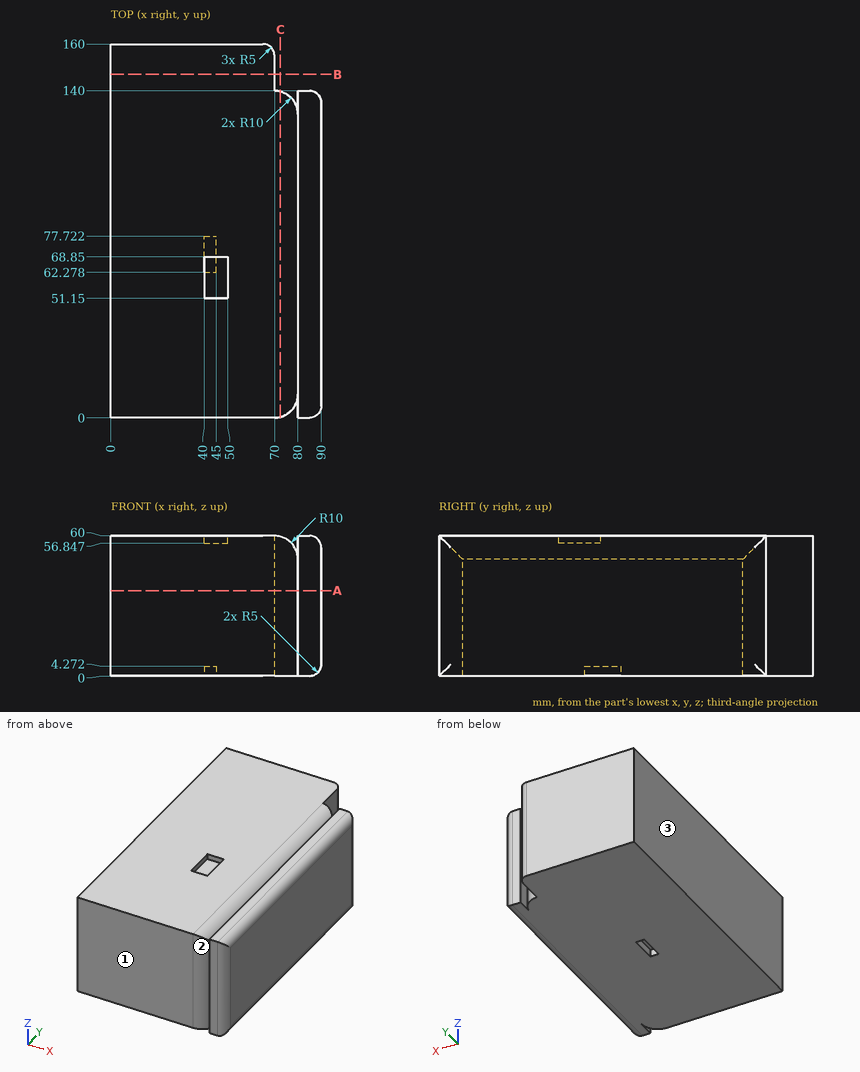
Answer from the drawing. Dimensions are ordinates in mm from the lowest x, y and z of the part. Give positions to 0.01 mm unless a question says otherwise; leave off trailing zeros. Order: outer loops, then holes, each group sorted by start corner. A loop starts at its lowest first (then second) coordinate and runs counter-clockwise, first axis right, second up. Notation, with made-up numbers: (2, 40.25) - (32, 40.25) arc R25 ccw to (32, 77.25) - close; hole circle Ø7 at (-34, 38). An arc over 180 degrees is marked (long way). One line per item, written item: value. Start each with the question number.
1. Section B-B, the plane y = 147 is taken. Write down the section's boundary in (x, z), then the cut area to 3 significant figures.
2. Each of these flat-tipped pins is pushed along its axis until it touches: pin 1 Ø1.5 at (x, z) = (83, 31) entering from +Y; pin 2 Ø2 at (y, z) = (70.5, 2.5) entering from +X; pin 3 Ø5 at (x, y) = (47, 64.5) entering from +Z. Where does it stop, or does it pass through?
3. Consider line 1 (X direction, y = 134.5, z = 38.5); line 2 (X direction, y = 149.5, z = 8); line 3 (X direction, y = 52, z = 53.5). Determine where each line is inside the solid, lowest interval first.
4. Section A-A, the plane z = 36.5 is taken. Write down the section's boundary in (x, y).
5. For a pull along X with two mould halves and no side action, classify the marked faces 1, 2 and 3 as released by +X, released by -X, zero draft, split by the parting line, or undercut.
6. Section C-C, the plane x = 72.5 is taken. Write down the section's boundary in (y, z).
Filled sheet:
1. outline: (0, 0) - (70, 0) - (70, 60) - (0, 60) - close
1. area: 4,200 mm²
2. pin 1: y = 140
2. pin 2: x = 89.77
2. pin 3: z = 56.85
3. line 1: 0 to 78.93, 80 to 90
3. line 2: 0 to 70
3. line 3: 0 to 79.37, 80 to 90
4. outline: (0, 0) - (70, 0) arc R10 ccw to (80, 10) - (80, 0) - (85, 0) arc R5 ccw to (90, 5) - (90, 135) arc R5 ccw to (85, 140) - (80, 140) - (80, 130) arc R10 ccw to (70, 140) - (70, 155) arc R5 ccw to (65, 160) - (0, 160) - close
5. face 1: zero draft
5. face 2: undercut
5. face 3: released by -X
6. outline: (0.32, 0) - (139.68, 0) - (139.68, 59.68) - (0.32, 59.68) - close
